from build123d import *

# Parameters (mm, degrees)
F0_R     = 11.05
F1_DEPTH = 8
F2_COUNT = 3
F3_R     = 10
F4_R     = 5
F5_SIZE  = 1


with BuildPart() as f1:
    # F0 (on Top) → F1 (new body)
    with BuildSketch(Plane.XY):
        with BuildLine():
            ThreePointArc((-12.6514260567, 23.6933629251), (-11.3751248169, 14.1917767316), (-13.1613477418, 4.7727272727))
            ThreePointArc((-13.1613477418, 4.7727272727), (-3.9842769003, -13.421085559), (13.6336360909, -3.1818181818))
            ThreePointArc((13.6336360909, -3.1818181818), (15.7271441431, 15), (13.6336360909, 33.1818181818))
            ThreePointArc((13.6336360909, 33.1818181818), (3.1856807408, 43.6327340698), (-10.8117310602, 38.8941818894))
            ThreePointArc((-10.8117310602, 38.8941818894), (-13.7694685953, 39.0065439815), (-16.6610679634, 38.374492037))
            ThreePointArc((-16.6610679634, 38.374492037), (-16.7251928987, 38.2586862032), (-16.6182205389, 38.1807124082))
            ThreePointArc((-16.6182205389, 38.1807124082), (-14.990242489, 38.1077523786), (-13.4439973475, 37.5932024207))
            ThreePointArc((-13.4439973475, 37.5932024207), (-12.4179647139, 35.2171421288), (-14.5954308534, 33.8181972809))
            ThreePointArc((-14.5954308534, 33.8181972809), (-16.7144110874, 34.3205676404), (-18.6910590274, 35.2345239477))
            ThreePointArc((-18.6910590274, 35.2345239477), (-18.82124029, 35.2092689611), (-18.8118896462, 35.0769906902))
            ThreePointArc((-18.8118896462, 35.0769906902), (-16.1822484317, 31.9388495716), (-14.2139807274, 28.3487430493))
            ThreePointArc((-14.2139807274, 28.3487430493), (-14.2850540536, 27.5953224844), (-14.9557406683, 27.2447894188))
            ThreePointArc((-14.9557406683, 27.2447894188), (-16.8849368279, 27.8185608598), (-18.2353559933, 29.311001668))
            ThreePointArc((-18.2353559933, 29.311001668), (-18.3566059607, 29.361220693), (-18.4231712091, 29.2481164368))
            ThreePointArc((-18.4231712091, 29.2481164368), (-16.9723331855, 26.5082159897), (-14.218759745, 25.0834989167))
            ThreePointArc((-14.218759745, 25.0834989167), (-13.2385127521, 24.6100687257), (-12.6514260567, 23.6933629251))
        make_face()
        Circle(F0_R, mode=Mode.SUBTRACT)
        with Locations((0, 30)):
            Circle(F0_R, mode=Mode.SUBTRACT)
    extrude(amount=F1_DEPTH)

    # F2: F1 ×3 about axis
    f2_axis = Axis((0, 0, 0), (0, 0, -1))


with BuildPart() as f1_1:
    add(f1.part)
    for i in range(1, F2_COUNT):
        add(f1.part.rotate(f2_axis, i * 360 / F2_COUNT))

    # F3
    f3_edges = [f1_1.edges().sort_by_distance(p)[0] for p in [
        (15.072251, 4.78462, 4),
        (-3.392523, -15.445263, 4),
        (-11.679728, 10.660642, 4),
    ]]
    fillet(f3_edges, radius=F3_R)

    # F4
    f4_edges = [f1_1.edges().sort_by_distance(p)[0] for p in [
        (-28.277484, -28.810325, 4),
        (39.089215, -10.083857, 4),
        (-10.811731, 38.894182, 4),
    ]]
    fillet(f4_edges, radius=F4_R)

    # F5
    f5_edges = [f1_1.edges().sort_by_distance(p)[0] for p in [
        (-11.05, 30, 8),
        (-11.05, 30, 0),
        (-11.05, 0, 8),
        (-11.05, 0, 0),
        (31.505762, -5.430419, 8),
        (31.505762, -5.430419, 0),
        (-20.455762, -24.569581, 8),
        (-20.455762, -24.569581, 0),
    ]]
    chamfer(f5_edges, length=F5_SIZE)


solid = f1_1.part
Check sheet for the modelled part. Datum: model origin and axes. Units: mm. A direction names the side the tool comes from. Give positions to 0.01 mm unless a question says otherwise; leave off trailing zeros. Loops run counter-clockwise (first coordinate to the right, second up) from the corner with the lowest first, then second, coordinate; pieces in that order, holes last. Notation, with made-up numbers: M 25.5,17 L 30.5,17 A13 cw 30.5,32 Z; hole C -4,-15.5 d5. An arc over 180 degrees is marked long. Answer as a JSON object with one key per item and string values. Group by question number.
Q1. Access from +Z, -Z, +X, -X, +Y, -Y to the whole of each face (thin tool, end or side, straight path). Record for faces 1 (the cylindrical face through (-14.7, -23.8, 3.9)), 2 (the flat face through (12, -3, 0)), 3 (the cylindrical face through (-12.218, -20.881, 3.944)), 4 (the cylindrical face through (-11.975, 21.021, 3.944)), 5 (the cylindrical face through (-26.315, -32.187, 3.944)).
Q2. Material ranges on line 1 along Y through (x, z) = (32.5, 2.25); line 2 along Y through (x, z) = (2, 5.25); line 3 along Y through (x, z) = (25, 1.5), recorded low to high. Write a range as [from, to].
Q3. Go/stop test with flat-tipped pins: P1, Ø12, axis at x = 28.5, y = -16.5, coming from the -Z side; P2, Ø4, axis at y = -23.5, z = 7, coming from the +X side; P3, Ø10, axis at x = 19.5, y = 4, coming from the +Z side; P4, Ø1.5, axis at y = -21.5, z = 4, coming from the +X side. Record where each tip stops, or that it passes through.
Q4. Cross-section at B-B on x = 0. Give the number of separate pieces and of enclosed holes in the cut face, then the cut area to 3 significant figures.
Q5. Release check for a two-part mould opening along Y. For faces 6 (the cylindrical face through (41.03, -6.7, 3.94)), 7 (the cylindrical face through (27.947, -0.835, 3.944)), 8 (the cylindrical face through (5.94, 39.32, 3.96)) record: released by +Y, released by -Y, zero draft, split by the parting line, or undercut.
Q6. Cross-section at A-A on y = -15. Record the cut outline in (x, z), then the cut area to 3 significant figures.
Evaluation:
{
 "1": {"face 1": "+Z, -Z", "face 2": "-Z, +X, -X, +Y, -Y", "face 3": "+Z, -Z, -Y", "face 4": "+Z, -Z, -X", "face 5": "+Z, -Z, -X, -Y"},
 "2": {"line 1": "y = [-27.39, -23.92], [-6.08, -1.95], [0.7, 1.62]", "line 2": "y = [-19.22, -10.87], [10.87, 19.13], [40.87, 43.86]", "line 3": "y = [-28.97, -26.01], [-3.99, -0.4]"},
 "3": {"P1": "passes through", "P2": "stops at x = 38.38", "P3": "stops at z = 8", "P4": "stops at x = 38.75"},
 "4": {"separate pieces": "3", "enclosed holes": "0", "area": "139 mm2"},
 "5": {"face 6": "released by -Y", "face 7": "released by +Y", "face 8": "undercut"},
 "6": {"outline": "M -39.98,0 L -38.03,0 L -37.03,1 L -37.03,7 L -38.03,8 L -39.98,8 Z; M -14.93,1 L -13.93,0 L 13.93,0 L 14.93,1 L 14.93,7 L 13.93,8 L -13.93,8 L -14.93,7 Z; M 37.03,1 L 38.03,0 L 39.98,0 L 39.98,8 L 38.03,8 L 37.03,7 Z", "area": "282 mm2"}
}
